from build123d import *

# Parameters (mm, degrees)
F0_R     = 2.7559
F1_DEPTH = 3.175


with BuildPart() as f1:
    # F0 (on Front) → F1 (new body)
    with BuildSketch(Plane.XZ):
        Polygon((1.1e-05, -14.514416), (1.1e-05, -40), (50.800011, -40), (50.800011, 0), (-20, 50.8), (-20, 0), (1.1e-05, 0), align=None)
        with Locations((16.933344, -29.999995)):
            Circle(F0_R, mode=Mode.SUBTRACT)
        with Locations((33.866677, -29.999995)):
            Circle(F0_R, mode=Mode.SUBTRACT)
        with Locations((16.933344, -10.000005)):
            Circle(F0_R, mode=Mode.SUBTRACT)
        with Locations((33.866677, -10.000005)):
            Circle(F0_R, mode=Mode.SUBTRACT)
        with Locations((-9.999995, 16.933333)):
            Circle(F0_R, mode=Mode.SUBTRACT)
        with Locations((10.000016, 8.907365)):
            Circle(F0_R, mode=Mode.SUBTRACT)
        with Locations((-9.999995, 33.866667)):
            Circle(F0_R, mode=Mode.SUBTRACT)
    extrude(amount=-F1_DEPTH)


solid = f1.part
Design review of the part built by this model. Coordinates are the model's own, in mm. A direction names the side the tool comes from. Round coordinates to 2 decimals unless told otherwise and drop trailing zeros. Write each loop counter-clockwise with the first axis right and the second up, starting at its lowest first coordinate (ties: lowest second). Pieces come first, ordered by that corner, then holes. Notation, with made-up numbers: (-14.75, -26) -> (33.25, -26) arc R7 ccw to (33.25, -17) -> close; hole circle Ø6 at (-40, -22.75). An arc over 180 degrees is marked (long way). One line per item, written item: value. Start each with the question number.
Q1. Insertion check: P1, Ø1.5, axis at x = 24, y = 2.5, coming from the +Z side; P2, Ø6.5, axis at x = 16.93, z = -30, coming from the -Y side; P3, Ø1, axis at x = -7.5, y = 1.5, coming from the -Z side. Each pin has a flat end and moves straight along its axis. Give the tip position at first contact, or say it passes through.
Q2. Add section B-B (x = 10). Give the boundary of the cut face in (y, z) (3 decimals), then the cut area to 3 significant figures.
Q3. Add section A-A (z = 18). Give the boundary of the cut face in (x, y) (3 decimals).
Q4. Add section C-C (y = 1.55). Give the boundary of the cut face in (x, z).
Q5. Tool access review of faces 5 (the face through (0, 2, -20)), 6 (the face through (25, 2, -40)): name each direction out of +Z, -Z, +X, -X, +Y, -Y from which nothing blocks a thin tool from reaching the whole face with its end or side.
Q6. Add section D-D (z = -23). Give the boundary of the cut face in (x, y) (3 decimals).
Q7. To check wall thickness, follow probe 1 along X at (y, z) = (1.1, -10.5); probe 2 along Z at (x, y) = (-10, 3.05); probe 3 along X at (y, z) = (1.9, -12). State the ranges of each line that lie inside material, in increasing order.
Q8. The part is to be moulded in two halves that separate along Z. For faces 1 (the face through (15, 3.175, -4)), 2 (the face through (-10, 2, 0)), 3 (the face through (-10.597, 1.565, 31.176)), 4 (the face through (15.9, 1.57, 25.04)), say which applies: pulls with the +Z half, pulls with the -Z half, needs draft (parallel to the pull), parting line crosses it, or undercut.
Response:
1. P1: stops at z = 19.77
1. P2: stops at y = 0
1. P3: stops at z = 0
2. outline: (0, -40) -> (3.175, -40) -> (3.175, 6.151) -> (0, 6.151) -> close; (0, 11.663) -> (3.175, 11.663) -> (3.175, 29.275) -> (0, 29.275) -> close
2. area: 202 mm^2
3. outline: (-20, 0) -> (-12.541, 0) -> (-12.541, 3.175) -> (-20, 3.175) -> close; (-7.459, 0) -> (25.713, 0) -> (25.713, 3.175) -> (-7.459, 3.175) -> close
4. outline: (-20, 0) -> (0, 0) -> (0, -40) -> (50.8, -40) -> (50.8, 0) -> (-20, 50.8) -> close; hole circle Ø5.51 at (-10, 16.93); hole circle Ø5.51 at (-10, 33.87); hole circle Ø5.51 at (10, 8.91); hole circle Ø5.51 at (16.93, -30); hole circle Ø5.51 at (16.93, -10); hole circle Ø5.51 at (33.87, -30); hole circle Ø5.51 at (33.87, -10)
5. face 5: -Z, -X, +Y, -Y
5. face 6: -Z, +X, -X, +Y, -Y
6. outline: (0, 0) -> (50.8, 0) -> (50.8, 3.175) -> (0, 3.175) -> close
7. probe 1: x = 0 to 14.22, 19.64 to 31.16, 36.58 to 50.8
7. probe 2: z = 0 to 14.18, 19.69 to 31.11, 36.62 to 43.62
7. probe 3: x = 0 to 15.04, 18.83 to 31.97, 35.76 to 50.8
8. face 1: needs draft
8. face 2: pulls with the -Z half
8. face 3: undercut
8. face 4: pulls with the +Z half
